Verification items for the finished model (mm, model axes). A direction names the side the tool comes from. Give positions to 0.01 mm unless a question says otherwise; leave off trailing zeros. Order: outer loops, then holes, each group sorted by start corner. A loop starts at its lowest first (then second) coordinate and runs counter-clockwise, first axis right, second up.
from build123d import *

# Parameters (mm, degrees)
PROFILE_LASER_PROFILE_3MM_R   = 2.2
PROFILE_LASER_PROFILE_3MM_R_2 = 0.9
PROFILE_LASER_PROFILE_3MM_W   = 3.1
PROFILE_LASER_PROFILE_3MM_H   = 3.1
PROFILE_LASER_PROFILE_3MM_W_2 = 6.1
LASER_PROFILE_3MM_DEPTH       = 3


with BuildPart() as part:
    # Profile_Laser_profile_3mm → Laser_profile_3mm (new body)
    with BuildSketch(Plane.XY):
        Polygon((0, 30.427227289), (8, 18), (4, 18), (12, 7), (10, 7), (14, -7), (10, -7), (14, -20), (10, -20), (14, -33), (4, -33), (4, -49.572772711), (-4, -49.572772711), (-4, -33), (-14, -33), (-10, -20), (-14, -20), (-10, -7), (-14, -7), (-10, 7), (-12, 7), (-4, 18), (-8, 18), align=None)
        Circle(PROFILE_LASER_PROFILE_3MM_R, mode=Mode.SUBTRACT)
        with Locations((0, -4.5)):
            Circle(PROFILE_LASER_PROFILE_3MM_R_2, mode=Mode.SUBTRACT)
        with Locations((0, 4.5)):
            Circle(PROFILE_LASER_PROFILE_3MM_R_2, mode=Mode.SUBTRACT)
        with Locations((-7.35, 3.5)):
            Rectangle(PROFILE_LASER_PROFILE_3MM_W, PROFILE_LASER_PROFILE_3MM_H, mode=Mode.SUBTRACT)
        with Locations((-7.35, -2.5)):
            Rectangle(PROFILE_LASER_PROFILE_3MM_W, PROFILE_LASER_PROFILE_3MM_H, mode=Mode.SUBTRACT)
        with Locations((-7.35, -25.5)):
            Rectangle(PROFILE_LASER_PROFILE_3MM_W, PROFILE_LASER_PROFILE_3MM_H, mode=Mode.SUBTRACT)
        with Locations((7.35, 3.5)):
            Rectangle(PROFILE_LASER_PROFILE_3MM_W, PROFILE_LASER_PROFILE_3MM_H, mode=Mode.SUBTRACT)
        with Locations((7.35, -2.5)):
            Rectangle(PROFILE_LASER_PROFILE_3MM_W, PROFILE_LASER_PROFILE_3MM_H, mode=Mode.SUBTRACT)
        with Locations((7.35, -25.5)):
            Rectangle(PROFILE_LASER_PROFILE_3MM_W, PROFILE_LASER_PROFILE_3MM_H, mode=Mode.SUBTRACT)
        with Locations((0, -10)):
            Rectangle(PROFILE_LASER_PROFILE_3MM_W_2, PROFILE_LASER_PROFILE_3MM_H, mode=Mode.SUBTRACT)
    extrude(amount=LASER_PROFILE_3MM_DEPTH)


solid = part.part
(1) Scan lines: line 1 (Y direction, x = -2, z = 1.45); line 2 (Y direction, x = -8.5, z = 0.9); line 3 (Y direction, x = 2.75, z = 2.85). Record each from-to range of solid material in increasing order.
Solved:
line 1: y = -49.57 to -11.55, -8.45 to -0.92, 0.92 to 27.32
line 2: y = -33 to -27.05, -23.95 to -4.05, -0.95 to 1.95, 5.05 to 11.81
line 3: y = -49.57 to -11.55, -8.45 to 26.16
(2) Section check B-B, the plane x = 6.5. Enter the section's corners in (y, z), then the cut area to 3 significant figures.
Solved:
outline: (-33, 0) - (-27.05, 0) - (-27.05, 3) - (-33, 3) - close; (-23.95, 0) - (-4.05, 0) - (-4.05, 3) - (-23.95, 3) - close; (-0.95, 0) - (1.95, 0) - (1.95, 3) - (-0.95, 3) - close; (5.05, 0) - (14.56, 0) - (14.56, 3) - (5.05, 3) - close; (18, 0) - (20.33, 0) - (20.33, 3) - (18, 3) - close
area: 122 mm2
(3) Go/stop test with flat-tipped pins: pin 1 (1.5 mm diameter, centred on y = 4, z = 1.5, fed in from -X); pin 2 (1.6 mm diameter, centred on x = 11, z = 2, fed in from -Y); pin 3 (1.5 mm diameter, centred on y = -26, z = 2, fed in from +X). Record where each tip stops, or that it passes through.
Solved:
pin 1: stops at x = -11.07
pin 2: stops at y = -33
pin 3: stops at x = 12.08
(4) Section check C-C, the plane x = 11.25. Enter the section's corners in (y, z) (1 decimal).
Solved:
outline: (-33, 0) - (-24.1, 0) - (-24.1, 3) - (-33, 3) - close; (-20, 0) - (-11.1, 0) - (-11.1, 3) - (-20, 3) - close; (-7, 0) - (2.6, 0) - (2.6, 3) - (-7, 3) - close; (7, 0) - (8, 0) - (8, 3) - (7, 3) - close
(5) Set-up check for faces 4 (the flat face through (8.9, 3, 1)), 5 (the flat face through (-12.028, -26.591, 1.479)), 6 (the flat face through (11.972, -13.409, 1.479)), 7 (the flat face through (3.944, 24.301, 1.479)): record each of +Z, -Z, +X, -X, +Y, -Y from which the full face is reachable in a straight line by a thin tool's end or side.
Solved:
face 4: +Z, -Z
face 5: +Z, -Z, -X
face 6: +Z, -Z, +X
face 7: +Z, -Z, +X, +Y
(6) Section check D-D, the plane z = 0.45. Give the number of separate pieces and of enclosed holes in the cut face, then the cut area to 3 significant figures.
Solved:
separate pieces: 1
enclosed holes: 10
area: 1,270 mm2
(7) Release check for a two-part mould opening along Y. For faces 1 (the flat face through (4, -41, 1)), 2 (the flat face through (-5.8, 3, 1)), 3 (the flat face through (-9, -33, 1)) record: pulls with the +Y half, pulls with the -Y half, needs draft (parallel to the pull), parting line crosses it, or undercut.
Solved:
face 1: needs draft
face 2: undercut
face 3: pulls with the -Y half
(8) Section check A-A, the plane x = -5. Enter the section's corners in (y, z) (3 decimals), then the cut area to 3 significant figures.
Solved:
outline: (-33, 0) - (16.625, 0) - (16.625, 3) - (-33, 3) - close; (18, 0) - (22.66, 0) - (22.66, 3) - (18, 3) - close
area: 163 mm2
